from build123d import *

# Parameters (mm, degrees)
SKETCH1_W           = 114
SKETCH1_H           = 40
SKETCH1_R           = 7.45
SKETCH1_R_2         = 9.525
BOSS_EXTRUDE1_DEPTH = 5.08
FILLET1_R           = 10
SKETCH2_R           = 3.175
SKETCH2_W           = 5.08
SKETCH2_H           = 20
CUT_EXTRUDE1_DEPTH  = 6.08


with BuildPart() as part:
    # Sketch1 → Boss-Extrude1 (new body)
    with BuildSketch(Plane(origin=(0, 0, 0), x_dir=(1, 0, 0), z_dir=(0, 1, 0))):
        Rectangle(SKETCH1_W, SKETCH1_H)
        with Locations((-45, 0)):
            Circle(SKETCH1_R, mode=Mode.SUBTRACT)
        with Locations((45, 0)):
            Circle(SKETCH1_R, mode=Mode.SUBTRACT)
        Circle(SKETCH1_R_2, mode=Mode.SUBTRACT)
    extrude(amount=BOSS_EXTRUDE1_DEPTH)

    # Fillet1
    fillet1_edges = [part.edges().sort_by_distance(p)[0] for p in [
        (-57, 2.54, -20),
        (57, 2.54, -20),
        (57, 2.54, 20),
        (-57, 2.54, 20),
    ]]
    fillet(fillet1_edges, radius=FILLET1_R)

    # Sketch2 → Cut-Extrude1 (cut, through all)
    with BuildSketch(Plane(origin=(0, 5.08, 0), x_dir=(1, 0, 0), z_dir=(0, 1, 0))):
        with Locations((10.75, -10.75)):
            Circle(SKETCH2_R)
        with Locations((-10.75, -10.75)):
            Circle(SKETCH2_R)
        with Locations((-10.75, 10.75)):
            Circle(SKETCH2_R)
        with Locations((10.75, 10.75)):
            Circle(SKETCH2_R)
        with Locations((-25.04, -10)):
            Rectangle(SKETCH2_W, SKETCH2_H)
        with Locations((25.04, -10)):
            Rectangle(SKETCH2_W, SKETCH2_H)
    extrude(amount=-CUT_EXTRUDE1_DEPTH, mode=Mode.SUBTRACT)


solid = part.part
Work out the finished part from the listing and answer in its coordinate system (mm). A direction names the side the tool comes from. Round coordinates to 2 decimals unless told otherwise and drop trailing zeros. Write each loop counter-clockwise with the first axis right and the second up, starting at its lowest first coordinate (ties: lowest second). Pieces come first, ordered by that corner, then holes. Notation, with made-up numbers: (50.25, 50.5) - (98.25, 50.5) arc R28 ccw to (98.25, 71.5) - close; hole circle Ø5 at (86, 49.25). An arc over 180 degrees is marked (long way). Answer in a Markdown table with one row per item. Add a question column.
1. Find the intervals of material crossed by line 1 along Z through (x, y) = (-10.75, 2.2) (3 decimals); line 2 along X through (y, z) = (4.25, 14); line 3 along Z through (x, y) = (-45, 2.55), in increasing order. Write a range as from..to.
2. A cutting plane is placed at D-D, the plane z = 3.5. Determine the outline of the cut face in (x, y).
3. A cutting plane is placed at C-C, the plane x = -45. Determine the outline of the cut face in (y, z), and give its area (3 significant figures).
4. A cutting plane is placed at A-A, the plane x = 10.75. Determine the outline of the cut face in (y, z) (3 decimals), and give its area (3 significant figures).
5. For faces 4 (the cylindrical face through (-50.912, 2.504, 4.533)), 5 (the flat face through (27.58, 3, 10)), determine the directions among +Z, -Z, +X, -X, +Y, -Y from which every point of the face is accessible in a straight line to the end or side of a thin tool.
6. Given pin 1 (1.5 mm diameter, centred on y = 3.5, z = 14.5, fed in from +X); pin 2 (1.5 mm diameter, centred on x = -25.5, y = 3.5, fed in from +Z), each flat-ended and moving along its own axis, determine where each tip first touches the part or whether it passes through.
7. The mould has two halves that part along Z. Classify faces 1 (the flat face through (-22.5, 3, 10)), 2 (the cylindrical face through (-7.72, 2.58, -11.7)), 3 (the flat face through (-1, 3, -20)): +Z half, -Z half, draft (parallel to the pull), parting line (faces both ways), or undercut.
8. A cutting plane is placed at B-B, the plane y = 2.45. Determine the outline of the cut face in (x, z) (3 decimals).
Worked out:
| question | item | result |
|---|---|---|
| 1 | line 1 | -20..-13.925, -7.575..7.575, 13.925..20 |
| 1 | line 2 | -56.17..-27.58, -22.5..22.5, 27.58..56.17 |
| 1 | line 3 | -20..-7.45, 7.45..20 |
| 2 | outline | (-57, 0) - (-51.58, 0) - (-51.58, 5.08) - (-57, 5.08) - close; (-38.42, 0) - (-27.58, 0) - (-27.58, 5.08) - (-38.42, 5.08) - close; (-22.5, 0) - (-8.86, 0) - (-8.86, 5.08) - (-22.5, 5.08) - close; (8.86, 0) - (22.5, 0) - (22.5, 5.08) - (8.86, 5.08) - close; (27.58, 0) - (38.42, 0) - (38.42, 5.08) - (27.58, 5.08) - close; (51.58, 0) - (57, 0) - (57, 5.08) - (51.58, 5.08) - close |
| 3 | outline | (0, -20) - (5.08, -20) - (5.08, -7.45) - (0, -7.45) - close; (0, 7.45) - (5.08, 7.45) - (5.08, 20) - (0, 20) - close |
| 3 | area | 128 mm^2 |
| 4 | outline | (0, -20) - (5.08, -20) - (5.08, -13.925) - (0, -13.925) - close; (0, -7.575) - (5.08, -7.575) - (5.08, 7.575) - (0, 7.575) - close; (0, 13.925) - (5.08, 13.925) - (5.08, 20) - (0, 20) - close |
| 4 | area | 139 mm^2 |
| 5 | face 4 | +Y, -Y |
| 5 | face 5 | +Z, +Y, -Y |
| 6 | pin 1 | x = 56.27 |
| 6 | pin 2 | z = 0 |
| 7 | face 1 | draft |
| 7 | face 2 | undercut |
| 7 | face 3 | -Z half |
| 8 | outline | (-57, -10) arc R10 ccw to (-47, -20) - (47, -20) arc R10 ccw to (57, -10) - (57, 10) arc R10 ccw to (47, 20) - (27.58, 20) - (27.58, 0) - (22.5, 0) - (22.5, 20) - (-22.5, 20) - (-22.5, 0) - (-27.58, 0) - (-27.58, 20) - (-47, 20) arc R10 ccw to (-57, 10) - close; hole circle Ø14.9 at (-45, 0); hole circle Ø6.35 at (-10.75, -10.75); hole circle Ø6.35 at (-10.75, 10.75); hole circle Ø19.05 at (0, 0); hole circle Ø6.35 at (10.75, -10.75); hole circle Ø6.35 at (10.75, 10.75); hole circle Ø14.9 at (45, 0) |
